Here's the drawing with two shaded views (mm, measured from the low corner). I have some questions. Give positions to 0.01 mm unless a question says otherwise; leave off trailing zeros. Write each loop counter-clockwise with the first axis right and the second up, starting at its lowest first coordinate (ties: lowest second). Pieces come first, ordered by that corner, then holes. Notation, with made-up numbers: (-26.5, 10.25) -> (-14.5, 10.25) arc R25 cw to (-14.5, 26.25) -> close; hole circle Ø11 at (72.5, -6). An arc over 180 degrees is marked (long way). One line per question, with ' | ' between items.
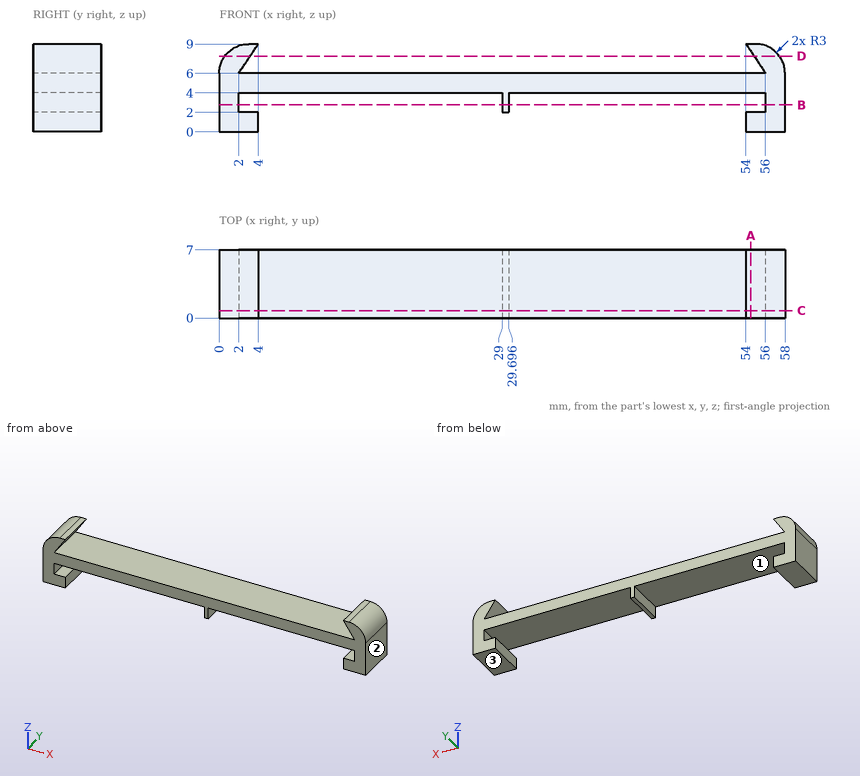
Q1. Imagine slicing it at A-A on x = 54.5. Please give me the cut outline in (y, z).
Answer below:
outline: (0, 0) -> (7, 0) -> (7, 2) -> (0, 2) -> close; (0, 4) -> (7, 4) -> (7, 6) -> (0, 6) -> close; (0, 8.25) -> (7, 8.25) -> (7, 9) -> (0, 9) -> close
Q2. Imagine slicing it at C-C on y = 0.75. Please give me the cut outline in (x, z), and give its area (3 significant figures).
Answer below:
outline: (0, 0) -> (4, 0) -> (4, 2) -> (2, 2) -> (2, 4) -> (29, 4) -> (29, 2) -> (29.7, 2) -> (29.7, 4) -> (56, 4) -> (56, 2) -> (54, 2) -> (54, 0) -> (58, 0) -> (58, 6) arc R3 ccw to (55, 9) -> (54, 9) -> (56, 6) -> (2, 6) -> (4, 9) -> (3, 9) arc R3 ccw to (0, 6) -> close | area: 156 mm^2
Q3. Imagine slicing it at B-B on z = 2.75. Please give me the cut outline in (x, y), and give its area (3 significant figures).
Answer below:
outline: (0, 0) -> (2, 0) -> (2, 7) -> (0, 7) -> close; (29, 0) -> (29.7, 0) -> (29.7, 7) -> (29, 7) -> close; (56, 0) -> (58, 0) -> (58, 7) -> (56, 7) -> close | area: 32.9 mm^2
Q4. If we mould it in two halves opening along X, with no side actions, what happens to the marked faces 1, 2 and 3? For each: +X half, -X half, draft (parallel to the pull), parting line (faces both ways), or undercut.
Answer below:
face 1: undercut | face 2: +X half | face 3: draft
Q5. Imagine slicing it at D-D on z = 7.75. Please give me the cut outline in (x, y).
Answer below:
outline: (0.56, 0) -> (3.17, 0) -> (3.17, 7) -> (0.56, 7) -> close; (54.83, 0) -> (57.44, 0) -> (57.44, 7) -> (54.83, 7) -> close
Q6. Will these pins go through, and if not, where does the flat tip stop? pin 1 (1 mm diameter, centred on x = 8, y = 2, fed in from -Z); pin 2 (1 mm diameter, centred on x = 2.5, y = 4, fed in from +Z); pin 3 (0.6 mm diameter, centred on x = 29.5, y = 3.5, fed in from -Z).
Answer below:
pin 1: stops at z = 4 | pin 2: stops at z = 9 | pin 3: stops at z = 2
Q7. If I drill on line 1 along X through (y, z) = (0.5, 1); line 2 along X through (y, z) = (4, 3.5); line 3 along Z through (x, y) = (3, 4.5), over which ranges is the centre line in solid material (lowest first)?
Answer below:
line 1: x = 0 to 4, 54 to 58 | line 2: x = 0 to 2, 29 to 29.7, 56 to 58 | line 3: z = 0 to 2, 4 to 6, 7.5 to 9
